from build123d import *

# Parameters (mm, degrees)
F0_R     = 3.7
F1_DEPTH = 25
F2_W     = 81.575442
F2_H     = 50.133398
F3_DEPTH = 18
F4_R     = 4.1
F4_R_2   = 0.75
F5_DEPTH = 16.001
F6_R     = 16
F7_DEPTH = 6


with BuildPart() as f1:
    # F0 (on Top) → F1 (new body)
    with BuildSketch(Plane.XY):
        with BuildLine():
            Line((-28, 3), (-28, 0))
            Line((-28, 0), (-28, -3))
            ThreePointArc((-28, -3), (-26.535534, -6.535534), (-23, -8))
            Line((-23, -8), (0, -8))
            Line((0, -8), (23, -8))
            ThreePointArc((23, -8), (26.535534, -6.535534), (28, -3))
            Line((28, -3), (28, 0))
            Line((28, 0), (28, 3))
            ThreePointArc((28, 3), (26.535534, 6.535534), (23, 8))
            Line((23, 8), (0, 8))
            Line((0, 8), (-23, 8))
            ThreePointArc((-23, 8), (-26.535534, 6.535534), (-28, 3))
        make_face()
        with Locations((-22, 0)):
            Circle(F0_R, mode=Mode.SUBTRACT)
        with Locations((22, 0)):
            Circle(F0_R, mode=Mode.SUBTRACT)
    extrude(amount=F1_DEPTH)

    # F2 (on face) → F3 (cut)
    with BuildSketch(Plane.XY.offset(25)):
        with Locations((1.883624, -0.796919)):
            Rectangle(F2_W, F2_H)
        Polygon((0, -3), (12, -3), (12, -8), (0, -8), (-12, -8), (-12, -3), align=None, mode=Mode.SUBTRACT)
        Polygon((12, 3), (0, 3), (-12, 3), (-12, 8), (0, 8), (12, 8), align=None, mode=Mode.SUBTRACT)
    extrude(amount=-F3_DEPTH, mode=Mode.SUBTRACT)

    # F4 (on face) → F5 (cut, through all)
    with BuildSketch(Plane.XZ.offset(8)):
        with Locations((0, 8)):
            Circle(F4_R)
        with Locations((-8.5, 8)):
            Circle(F4_R_2)
        with Locations((8.5, 8)):
            Circle(F4_R_2)
        with BuildLine():
            Line((-15.281343, 8), (-12, 8))
            ThreePointArc((-12, 8), (0, 20), (12, 8))
            Line((12, 8), (15.281343, 8))
            Line((15.281343, 8), (15.281343, 26.349186))
            Line((15.281343, 26.349186), (0, 26.349186))
            Line((0, 26.349186), (-15.281343, 26.349186))
            Line((-15.281343, 26.349186), (-15.281343, 8))
        make_face()
    extrude(amount=-F5_DEPTH, mode=Mode.SUBTRACT)

    # F6 (on face) → F7 (cut)
    with BuildSketch(Plane(origin=(0, -3, 0), x_dir=(-1, 0, 0), z_dir=(0, 1, 0))):
        with Locations((0, 8)):
            Circle(F6_R)
    extrude(amount=F7_DEPTH, mode=Mode.SUBTRACT)


solid = f1.part
Design review of the part built by this model. Coordinates are the model's own, in mm. A direction names the side the tool comes from. Coordinates: 2 decimals unless noted, no trailing zeros. Order: outer loops, then holes, each group sorted by start corner. A loop starts at its lowest first (then second) coordinate and runs counter-clockwise, first axis right, second up. Notation, with made-up numbers: (31, 25.25) - (85, 25.25) arc R24 ccw to (85, 52.25) - close; hole circle Ø7 at (-11, -16.5). An arc over 180 degrees is marked (long way). Put each result on its own line as item: value.
1) Wall thickness on L1, parallel to Y at x = 9, z = 2.25; L2, parallel to Y at x = 22, z = 4; L3, parallel to X at y = 0, z = 4.5: over which ranges is each line inside the solid? List them lowest first. Write a range as from..to.
Response values:
L1: y = -8..-3, 3..8
L2: y = -8..-3.7, 3.7..8
L3: x = -28..-25.7, -18.3..-15.61, 15.61..18.3, 25.7..28
2) Tool access review of faces 1 (the face through (27, 6, 3)), 2 (the face through (7.75, 5.46, 8.03)), 3 (the face through (15.333, -0.042, 3.427)), 4 (the face through (-12, -5.5, 7.5)), 5 (the face through (12, 5.5, 7.5)): name each direction out of +Z, -Z, +X, -X, +Y, -Y from which nothing blocks a thin tool from reaching the whole face with its end or side.
Response values:
face 1: +Z, -Z, +X, +Y
face 2: +Y, -Y
face 3: +Z
face 4: +Z, -X, +Y, -Y
face 5: +Z, +X, +Y, -Y
3) Take a section at D-D, the plane y = 6. Give the boundary of the cut face in (x, z), and give its area (3 significant figures).
Response values:
outline: (-27, 0) - (27, 0) - (27, 7) - (12, 7) - (12, 8) arc R12 ccw to (-12, 8) - (-12, 7) - (-27, 7) - close; hole circle Ø1.5 at (-8.5, 8); hole circle Ø8.2 at (0, 8); hole circle Ø1.5 at (8.5, 8)
area: 572 mm²
4) Take a section at C-C, the plane x = -8.5. Give the boundary of the cut face in (y, z), and give its area (3 significant figures).
Response values:
outline: (-8, 0) - (-3, 0) - (-3, 7.25) - (-8, 7.25) - close; (-8, 8.75) - (-3, 8.75) - (-3, 16.47) - (-8, 16.47) - close; (3, 0) - (8, 0) - (8, 7.25) - (3, 7.25) - close; (3, 8.75) - (8, 8.75) - (8, 16.47) - (3, 16.47) - close
area: 150 mm²
5) Insertion check: P1, Ø5, axis at x = -20, y = 3.5, coming from the +Z side; P2, Ø4, axis at y = 3, z = 9.5, coming from the +X side; P3, Ø0.8, axis at y = -4.5, z = 7.5, coming from the -X side; P4, Ø6, axis at x = 22, y = 0, coming from the +Z side. Each pin has a flat end and moves straight along its axis. Give the tip position at first contact, or say it passes through.
Response values:
P1: stops at z = 7
P2: stops at x = 12
P3: stops at x = -12
P4: passes through
6) The part is to be moulded in two halves that separate along Y. For faces 6 (the face through (-28, 0, 3)), 7 (the face through (-15.303, -0.042, 3.328)), 8 (the face through (0, -8, 3)), say which applies: released by +Y, released by -Y, zero draft, split by the parting line, or undercut.
Response values:
face 6: zero draft
face 7: undercut
face 8: released by -Y
7) Take a section at B-B, the plane x = -22. Give the boundary of the cut face in (y, z).
Response values:
outline: (-8, 0) - (-3.7, 0) - (-3.7, 7) - (-8, 7) - close; (3.7, 0) - (8, 0) - (8, 7) - (3.7, 7) - close
8) Take a section at A-A, the plane y = 0. Give the boundary of the cut face in (x, z).
Response values:
outline: (-28, 0) - (-25.7, 0) - (-25.7, 7) - (-28, 7) - close; (-18.3, 0) - (-13.86, 0) arc R16 cw to (-15.97, 7) - (-18.3, 7) - close; (13.86, 0) - (18.3, 0) - (18.3, 7) - (15.97, 7) arc R16 cw to start; (25.7, 0) - (28, 0) - (28, 7) - (25.7, 7) - close
